Could you check a few things on this drawing? It's one solid part, dimensions in mm from its lowest x, y, z. Give positions to 0.01 mm unless a question says otherwise; leave off trailing zeros. Write each loop counter-clockwise with the first axis right and the second up, starting at its lowest first coordinate (ties: lowest second). Pieces come first, ordered by that corner, then holes. Notation, with made-up numbers: M 60.25,5.25 L 83.25,5.25 A27 cw 83.25,39.25 Z; hole C 33.25,31 d5. An arc over 180 degrees is marked long. Write each question's results on one line, items separated by ' | '.
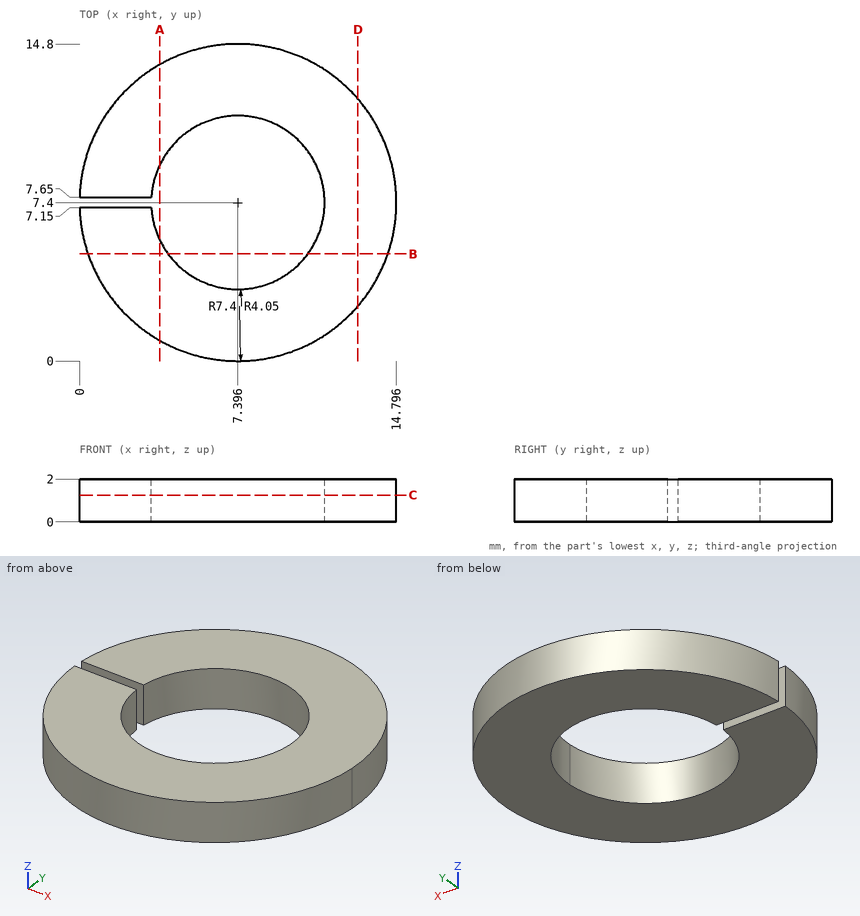
Item 1: I want a section at A-A, the plane x = 3.75. Please give me the cut outline in (y, z), and give its area (3 significant figures).
Geometry says:
outline: M 0.96,0 L 5.64,0 L 5.64,2 L 0.96,2 Z; M 9.16,0 L 13.84,0 L 13.84,2 L 9.16,2 Z | area: 18.7 mm2
Item 2: I want a section at C-C, the plane z = 1.25. Please give me the cut outline in (x, y), and give its area (3 significant figures).
Geometry says:
outline: M 0,7.15 A7.4 ccw long 0,7.65 L 3.35,7.65 A4.05 cw long 3.35,7.15 Z | area: 119 mm2
Item 3: I want a section at D-D, the plane x = 13. Please give me the cut outline in (y, z), and give its area (3 significant figures).
Geometry says:
outline: M 2.57,0 L 12.23,0 L 12.23,2 L 2.57,2 Z | area: 19.3 mm2
Item 4: I want a section at B-B, the plane y = 5. Please give me the cut outline in (x, z).
Geometry says:
outline: M 0.4,0 L 4.13,0 L 4.13,2 L 0.4,2 Z; M 10.66,0 L 14.4,0 L 14.4,2 L 10.66,2 Z
Item 5: If I drill on line 1 (X direction, y = 7.5, z = 1.3) (1 decimal); line 2 (X direction, y = 9, z = 1.6) (1 decimal); line 3 (X direction, y = 5, z = 1.05) (1 decimal), over which ranges is the centre line in solid material (lowest first)? Write a range as from..to.
Geometry says:
line 1: x = 11.4..14.8 | line 2: x = 0.2..3.7, 11.1..14.6 | line 3: x = 0.4..4.1, 10.7..14.4
Item 6: I'm going to push flat-ended pins straight in: pin 1 (1 mm diameter, centred on x = 2, z = 1, fed in from -Y); pin 2 (0.6 mm diameter, centred on x = 1, z = 1, fed in from +Y) (1 decimal). Where does each tip first touch, or does it pass through?
Geometry says:
pin 1: stops at y = 1.85 | pin 2: stops at y = 11.6
